```python
from build123d import *

# Parameters (mm, degrees)
SKETCH1_R           = 1.7
BOSS_EXTRUDE1_DEPTH = 6
CUT_EXTRUDE1_DEPTH  = 5


with BuildPart() as part:
    # Sketch1 → Boss-Extrude1 (new body)
    with BuildSketch(Plane(origin=(0, 0, 0), x_dir=(1, 0, 0), z_dir=(0, 1, 0))):
        with BuildLine():
            Line((-12, 0), (-12, 40))
            ThreePointArc((-12, 40), (0, 52), (12, 40))
            Line((12, 40), (12, 0))
            ThreePointArc((12, 0), (0, -12), (-12, 0))
        make_face()
        with Locations((0, 40)):
            Circle(SKETCH1_R, mode=Mode.SUBTRACT)
        Circle(SKETCH1_R, mode=Mode.SUBTRACT)
    extrude(amount=BOSS_EXTRUDE1_DEPTH)

    # Sketch2 → Cut-Extrude1 (cut)
    with BuildSketch(Plane(origin=(0, 6, 0), x_dir=(1, 0, 0), z_dir=(0, 1, 0))):
        Polygon((1.303325688, 12.608472723), (7.052913238, 17.432949516), (5.749587551, 24.824476793), (-1.303325688, 27.391527277), (-7.052913238, 22.567050484), (-5.749587551, 15.175523207), align=None)
    extrude(amount=-CUT_EXTRUDE1_DEPTH, mode=Mode.SUBTRACT)


solid = part.part
```
Input: part model. Units: mm. Frame: model coordinates. A direction names the side the tool comes from. Give positions to 0.01 mm unless a question says otherwise; leave off trailing zeros. Order: outer loops, then holes, each group sorted by start corner. A loop starts at its lowest first (then second) coordinate and runs counter-clockwise, first axis right, second up.
1. Cut plane D-D (z = -19.5). Return loops of the section in (x, y), and give its area (3 significant figures).
Computed:
outline: (-12, 0) - (12, 0) - (12, 6) - (6.69, 6) - (6.69, 1) - (-6.51, 1) - (-6.51, 6) - (-12, 6) - close
area: 78.0 mm2
2. Pin query (flat end, axial travel): pin 1 Ø3 at (x, y) = (8, 3.5) entering from +Z; pin 2 Ø1.5 at (x, y) = (-1, 5.5) entering from +Z. Return the tip coordinate at first contact, or that it passes through.
Computed:
pin 1: stops at z = 10.09
pin 2: stops at z = 12
3. Draft query along Z for faces 3 (the face through (-0.37, 2.96, -38.34)), 4 (the face through (0, 0, -20)), 5 (the face through (0, 3, 12)), 6 (the face through (0, 3, -52)). Return one class per face: released by +Z, released by -Z, zero draft, split by the parting line, or undercut.
Computed:
face 3: undercut
face 4: zero draft
face 5: released by +Z
face 6: released by -Z
4. Set-up query: faces 1 (the face through (-4.14, 3.54, -25.01)), 2 (the face through (0, 6, -28)). Return all of +Z, -Z, +X, -X, +Y, -Y with unobstructed straight access to the full face (end or side cutting, diameter ignored); none if empty.
Computed:
face 1: +Y
face 2: +Z, -Z, +X, -X, +Y
5. Line query: probe 1 along X at (y, z) = (4.75, -40); probe 2 along Z at (x, y) = (1, 1.25); probe 3 along Z at (x, y) = (0, 4.15). Output: solid intervals per line, ascending.
Computed:
probe 1: x = -12 to -1.7, 1.7 to 12
probe 2: z = -51.96 to -41.37, -38.63 to -26.55, -12.72 to -1.37, 1.37 to 11.96
probe 3: z = -52 to -41.7, -38.3 to -26.92, -13.08 to -1.7, 1.7 to 12
6. Cut plane B-B (x = 0). Return loops of the section in (y, z), and give its area (3 significant figures).
Computed:
outline: (0, -52) - (6, -52) - (6, -41.7) - (0, -41.7) - close; (0, -38.3) - (6, -38.3) - (6, -26.92) - (1, -26.92) - (1, -13.08) - (6, -13.08) - (6, -1.7) - (0, -1.7) - close; (0, 1.7) - (6, 1.7) - (6, 12) - (0, 12) - close
area: 274 mm2
7. Cut plane C-C (x = -4.5). Return loops of the section in (y, z), and give its area (3 significant figures).
Computed:
outline: (0, -51.12) - (6, -51.12) - (6, -24.71) - (1, -24.71) - (1, -14.72) - (6, -14.72) - (6, 11.12) - (0, 11.12) - close
area: 324 mm2
8. Cut plane A-A (y = 3.1). Return loops of the section in (x, z), and give its area (3 significant figures).
Computed:
outline: (-12, -40) arc R12 ccw to (12, -40) - (12, 0) arc R12 ccw to (-12, 0) - close; hole (-7.05, -22.57) - (-1.3, -27.39) - (5.75, -24.82) - (7.05, -17.43) - (1.3, -12.61) - (-5.75, -15.18) - close; hole circle Ø3.4 at (0, -40); hole circle Ø3.4 at (0, 0)
area: 1,250 mm2
